CAD build for the part. Positions are in the model's coordinates, mm. A direction names the side the tool comes from. Round coordinates to 2 decimals unless told otherwise and drop trailing zeros. Write each loop counter-clockwise with the first axis right and the second up, starting at its lowest first coordinate (ties: lowest second). Pieces come first, ordered by that corner, then holes. Notation, with made-up numbers: (-25.5, 85.5) - (-4.5, 85.5) arc R18 cw to (-4.5, 120.5) - close; hole circle Ø6 at (37.5, -2.75). An arc over 180 degrees is marked (long way). Answer in a Markdown table with one row per item.
```python
from build123d import *

# Parameters (mm, degrees)
SKETCH1_R           = 165.1
SKETCH1_R_2         = 3
BOSS_EXTRUDE1_DEPTH = 12.7
SKETCH7_R           = 165.1
SKETCH7_R_2         = 3
BOSS_EXTRUDE3_DEPTH = 6.35
SKETCH8_R           = 25
CUT_EXTRUDE1_DEPTH  = 6.35
CUT_EXTRUDE2_START  = -6.35
SKETCH9_R           = 25
CUT_EXTRUDE2_DEPTH  = 6.35
SKETCH10_R          = 165.1
CUT_EXTRUDE3_DEPTH  = 6.35
CUT_EXTRUDE5_START  = -3.175
SKETCH11_R          = 25
CUT_EXTRUDE5_DEPTH  = 3.175
BOSS_EXTRUDE4_START = 3.175
SKETCH12_R          = 25
BOSS_EXTRUDE4_DEPTH = 3.175
SKETCH13_R          = 3
CUT_EXTRUDE6_DEPTH  = 3.175


with BuildPart() as part:
    # Sketch1 → Boss-Extrude1 (new body)
    with BuildSketch(Plane(origin=(0, 0, 0), x_dir=(1, 0, 0), z_dir=(0, 1, 0))):
        with Locations(Location((0, 0, 0), (0, 0, 270))):
            Circle(SKETCH1_R)
        with Locations(Location((0, 0, 0), (0, 0, 270))):
            Circle(SKETCH1_R_2, mode=Mode.SUBTRACT)
    extrude(amount=BOSS_EXTRUDE1_DEPTH)

    # Sketch7 → Boss-Extrude3 (add)
    with BuildSketch(Plane(origin=(0, 12.7, 0), x_dir=(1, 0, 0), z_dir=(0, 1, 0))):
        with Locations(Location((0, 0, 0), (0, 0, 270))):
            Circle(SKETCH7_R)
        with Locations(Location((0, 0, 0), (0, 0, 270))):
            Circle(SKETCH7_R_2, mode=Mode.SUBTRACT)
    extrude(amount=BOSS_EXTRUDE3_DEPTH)

    # Sketch8 → Cut-Extrude1 (cut)
    with BuildSketch(Plane(origin=(0, 19.05, 0), x_dir=(1, 0, 0), z_dir=(0, 1, 0))):
        with Locations(Location((0, 0, 0), (0, 0, 270))):
            Circle(SKETCH8_R)
    extrude(amount=-CUT_EXTRUDE1_DEPTH, mode=Mode.SUBTRACT)

    # Sketch9 → Cut-Extrude2 (cut)
    with BuildSketch(Plane.XZ.offset(CUT_EXTRUDE2_START)):
        with Locations(Location((0, 0, 0), (0, 0, 90))):
            Circle(SKETCH9_R)
    extrude(amount=CUT_EXTRUDE2_DEPTH, mode=Mode.SUBTRACT)

    # Sketch10 → Cut-Extrude3 (cut)
    with BuildSketch(Plane.XZ):
        with Locations(Location((0, 0, 0), (0, 0, 270))):
            Circle(SKETCH10_R)
    extrude(amount=-CUT_EXTRUDE3_DEPTH, mode=Mode.SUBTRACT)

    # Sketch11 → Cut-Extrude5 (cut)
    with BuildSketch(Plane.XZ.offset(-6.35).offset(CUT_EXTRUDE5_START)):
        with Locations(Location((0, 0, 0), (0, 0, 90))):
            Circle(SKETCH11_R)
    extrude(amount=CUT_EXTRUDE5_DEPTH, mode=Mode.SUBTRACT)

    # Sketch12 → Boss-Extrude4 (add)
    with BuildSketch(Plane(origin=(0, 12.7, 0), x_dir=(1, 0, 0), z_dir=(0, 1, 0)).offset(BOSS_EXTRUDE4_START)):
        with Locations(Location((0, 0, 0), (0, 0, 270))):
            Circle(SKETCH12_R)
    extrude(amount=-BOSS_EXTRUDE4_DEPTH)

    # Sketch13 → Cut-Extrude6 (cut)
    with BuildSketch(Plane.XZ.offset(-12.7)):
        with Locations(Location((0, 0, 0), (0, 0, 270))):
            Circle(SKETCH13_R)
    extrude(amount=-CUT_EXTRUDE6_DEPTH, mode=Mode.SUBTRACT)


solid = part.part
```
Q1. Saw through at B-B on z = 145. List the corners of the cut face in (x, y).
Computed:
| item | result |
|---|---|
| outline | (-78.95, 6.35) - (78.95, 6.35) - (78.95, 19.05) - (-78.95, 19.05) - close |
Q2. Saw through at A-A on x = 42. List the corners of the cut face in (y, z).
Computed:
| item | result |
|---|---|
| outline | (6.35, -159.67) - (19.05, -159.67) - (19.05, 159.67) - (6.35, 159.67) - close |
Q3. 3-axis set-ups, long thin cutter, end or side, ignore diameter. For faces 4 (the flat face through (-5, 15.875, 0)), 5 (the cylindrical face through (-7.509, 7.96, 23.846)), 6 (the flat face through (-34, 6.35, 2)): which of +Z, -Z, +X, -X, +Y, -Y reach the whole face in a straight line?
Computed:
| item | result |
|---|---|
| face 4 | +Y |
| face 5 | -Y |
| face 6 | +Z, -Z, +X, -X, -Y |
Q4. Pull direction Z, two halves, no side cores. Call faces 1 (the cylindrical face through (7.509, 17.485, 23.846)), 2 (the flat face through (-34, 19.05, -2)), 3 (the cylindrical face through (163.695, 12.611, -21.493)): released by +Z, released by -Z, zero draft, split by the parting line, or undercut.
Computed:
| item | result |
|---|---|
| face 1 | undercut |
| face 2 | zero draft |
| face 3 | split by the parting line |
Q5. Drill centre lines: line 1 (X direction, y = 7.9, z = 0); line 2 (X direction, y = 17.75, z = -17.5); line 3 (Z direction, x = 8, y = 16). Where is each one in solid material? Low to high.
Computed:
| item | result |
|---|---|
| line 1 | x = -165.1 to -25, 25 to 165.1 |
| line 2 | x = -164.17 to -17.85, 17.85 to 164.17 |
| line 3 | z = -164.91 to -23.69, 23.69 to 164.91 |
Q6. Flat gauge pins, fed straight in: pin 1 (5 mm diameter, centred on x = 0, z = 0, fed in from +Y); pin 2 (1 mm diameter, centred on x = 89, y = 9, fed in from +Z); pin 3 (2 mm diameter, centred on y = 8, z = -79.5, fed in from -X); pin 4 (2 mm diameter, centred on y = 7.5, z = 8.5, fed in from -X). Where does each tip first touch, or does it go through?
Computed:
| item | result |
|---|---|
| pin 1 | passes through |
| pin 2 | stops at z = 139.38 |
| pin 3 | stops at x = -145.24 |
| pin 4 | stops at x = -164.93 |
